Model file for the job. Use its own axes, mm. Round coordinates to 2 decimals unless told otherwise and drop trailing zeros. Loops run counter-clockwise (first coordinate to the right, second up) from the corner with the lowest first, then second, coordinate; pieces in that order, holes last.
from build123d import *

# Parameters (mm, degrees)
SKETCH_1_R               = 56.85
SKETCH_1_R_2             = 44.35
EXTRUDE_1_DEPTH          = 4.275
CHAMFER_1_SIZE           = 0.5
SKETCH_2_R               = 2.5
CUT_EXTRUDE_1_DEPTH      = 10
PATTERN_CIRCULAR_1_COUNT = 4


with BuildPart() as part:
    # ｽｹｯﾁ1 → ﾎﾞｽ - 押し出し1 (new, symmetric)
    with BuildSketch(Plane(origin=(0, 0, 0), x_dir=(1, 0, 0), z_dir=(0, 1, 0))):
        with Locations(Location((0, 0, 0), (0, 0, 270))):
            Circle(SKETCH_1_R)
        with Locations(Location((0, 0, 0), (0, 0, 270))):
            Circle(SKETCH_1_R_2, mode=Mode.SUBTRACT)
    extrude(amount=EXTRUDE_1_DEPTH, both=True)

    # 面取り1
    chamfer_1_edges = [part.edges().sort_by_distance(p)[0] for p in [
        (0, -4.275, -56.85),
        (0, 4.275, -56.85),
        (0, -4.275, -44.35),
        (0, 4.275, -44.35),
    ]]
    chamfer(chamfer_1_edges, length=CHAMFER_1_SIZE)

    # ｽｹｯﾁ2 → ｶｯﾄ - 押し出し1 (cut)
    with BuildSketch(Plane(origin=(0, 4.275, 0), x_dir=(1, 0, 0), z_dir=(0, 1, 0))):
        with Locations(Location((0, 50.5, 0), (0, 0, 270))):
            Circle(SKETCH_2_R)
    extrude(amount=-CUT_EXTRUDE_1_DEPTH, mode=Mode.SUBTRACT)

    # ｽｹｯﾁ3 → M5 丸皿ねじ用皿穴1 (revolve, cut)
    with BuildSketch(Plane(origin=(0, 4.275, -50.5), x_dir=(0, 0, 1), z_dir=(1, 0, 0))):
        Polygon((0, 0), (0, 11.652366702), (2.75, 10), (2.75, 2.45), (5.2, 0), align=None)
    hole_wizard_m5_1 = revolve(axis=Axis((0, 10.625, -50.5), (0, -1, 0)), mode=Mode.SUBTRACT)

    # 円形ﾊﾟﾀｰﾝ1: M5 丸皿ねじ用皿穴1 ×4 about axis
    pattern_circular_1_axis = Axis((0, 0, 0), (0, 1, 0))
    for i in range(1, PATTERN_CIRCULAR_1_COUNT):
        add(hole_wizard_m5_1.rotate(pattern_circular_1_axis, i * 360 / PATTERN_CIRCULAR_1_COUNT), mode=Mode.SUBTRACT)


solid = part.part
Q1. Pull direction Z, two halves, no side cores. Call faces 1 (the face through (-34.592, 0.053, -45.114)), 2 (the face through (-25, 4.275, -38)), 3 (the face through (-1.112, 1.978, 47.818)): pulls with the +Z half, pulls with the -Z half, needs draft (parallel to the pull), parting line crosses it, or undercut.
Q2. Slice it at A-A on x = 0. Give the cut face in (y, z) (3 decimals), plus the area to 3 significant figures.
Q3. Slice it at B-B on z = 0. Give the cut face in (x, y) (3 decimals).
Q4. Flat gauge pins, fed straight in: P1, Ø2, axis at x = 14, y = 2, coming from the +Z side; P2, Ø6.5, axis at x = 0, z = -50.5, coming from the +Y side (3 decimals); P3, Ø1, axis at x = -29, y = -2.5, coming from the +Z side; P4, Ø9, axis at x = 0, z = 50.5, coming from the -Y side (3 decimals). Where does each tip first touch, or does it go through?
Q5. Slice it at C-C on y = -1. Give the cut face in (x, z).
Q6. Probe line 1 (Z direction, x = -3, y = -3.5); line 2 (Z direction, x = -26, y = 2.75); line 3 (X direction, y = -1.25, z = -5). List the from-to ranges inside material, lowest first.
Reply:
1. face 1: parting line crosses it
1. face 2: needs draft
1. face 3: undercut
2. outline: (-4.275, -56.35) - (-3.775, -56.85) - (3.775, -56.85) - (4.275, -56.35) - (4.275, -55.7) - (1.825, -53.25) - (-4.275, -53.25) - close; (-4.275, -47.75) - (1.825, -47.75) - (4.275, -45.3) - (4.275, -44.85) - (3.775, -44.35) - (-3.775, -44.35) - (-4.275, -44.85) - close; (-4.275, 44.85) - (-3.775, 44.35) - (3.775, 44.35) - (4.275, 44.85) - (4.275, 45.3) - (1.825, 47.75) - (-4.275, 47.75) - close; (-4.275, 53.25) - (1.825, 53.25) - (4.275, 55.7) - (4.275, 56.35) - (3.775, 56.85) - (-3.775, 56.85) - (-4.275, 56.35) - close
2. area: 107 mm2
3. outline: (-56.85, -3.775) - (-56.35, -4.275) - (-53.25, -4.275) - (-53.25, 1.825) - (-55.7, 4.275) - (-56.35, 4.275) - (-56.85, 3.775) - close; (-47.75, -4.275) - (-44.85, -4.275) - (-44.35, -3.775) - (-44.35, 3.775) - (-44.85, 4.275) - (-45.3, 4.275) - (-47.75, 1.825) - close; (44.35, -3.775) - (44.85, -4.275) - (47.75, -4.275) - (47.75, 1.825) - (45.3, 4.275) - (44.85, 4.275) - (44.35, 3.775) - close; (53.25, -4.275) - (56.35, -4.275) - (56.85, -3.775) - (56.85, 3.775) - (56.35, 4.275) - (55.7, 4.275) - (53.25, 1.825) - close
4. P1: stops at z = 55.34
4. P2: stops at y = 2.325
4. P3: stops at z = 49.19
4. P4: stops at y = -4.275
5. outline: circle Ø113.7 at (0, 0); hole circle Ø5.5 at (-50.5, 0); hole circle Ø88.7 at (0, 0); hole circle Ø5.5 at (0, -50.5); hole circle Ø5.5 at (0, 50.5); hole circle Ø5.5 at (50.5, 0)
6. line 1: z = -56.77 to -44.25, 44.25 to 56.77
6. line 2: z = -50.56 to -35.93, 35.93 to 50.56
6. line 3: x = -56.63 to -44.07, 44.07 to 56.63
